from build123d import *

# Parameters (mm, degrees)
SKETCH1_W              = 50
SKETCH1_H              = 50
BOSS_EXTRUDE1_DEPTH    = 6.35
SKETCH6_W              = 25.4
SKETCH6_H              = 25.4
BOSS_EXTRUDE3_DEPTH    = 12.7
SKETCH10_W             = 25.4
SKETCH10_H             = 25.4
CUT_EXTRUDE2_DEPTH     = 15.875
FILLET3_R              = 2.54
SKETCH11_W             = 9.125
SKETCH11_H             = 7.62
BOSS_EXTRUDE4_DEPTH    = 6.35
FILLET4_R              = 2.54
CUT_EXTRUDE3_DEPTH     = 7.35
FILLET4_OF_MIRROR1_R   = 2.54
FILLET5_R              = 2.54
CUT_EXTRUDE4_DEPTH     = 2.54
SKETCH14_R             = 4.7625
CUT_EXTRUDE5_DEPTH     = 16.875
FILLET6_R              = 2.54
F_10_CLEARANCE_HOLE1_D = 5.1054
F_8_CLEARANCE_HOLE1_D  = 4.4958


with BuildPart() as part:
    # Sketch1 → Boss-Extrude1 (new body)
    with BuildSketch(Plane.XY):
        Rectangle(SKETCH1_W, SKETCH1_H)
    extrude(amount=BOSS_EXTRUDE1_DEPTH)

    # Sketch6 → Boss-Extrude3 (add)
    with BuildSketch(Plane.XY.offset(6.35)):
        with BuildLine():
            Line((15.875, 19.05), (15.875, 25))
            Line((15.875, 25), (-15.875, 25))
            Line((-15.875, 25), (-15.875, 19.05))
            ThreePointArc((-15.875, 19.05), (-16.80493597, 16.80493597), (-19.05, 15.875))
            Line((-19.05, 15.875), (-25, 15.875))
            Line((-25, 15.875), (-25, -15.875))
            Line((-25, -15.875), (-19.05, -15.875))
            ThreePointArc((-19.05, -15.875), (-16.80493597, -16.80493597), (-15.875, -19.05))
            Line((-15.875, -19.05), (-15.875, -25))
            Line((-15.875, -25), (15.875, -25))
            Line((15.875, -25), (15.875, -19.05))
            ThreePointArc((15.875, -19.05), (16.80493597, -16.80493597), (19.05, -15.875))
            Line((19.05, -15.875), (25, -15.875))
            Line((25, -15.875), (25, 15.875))
            Line((25, 15.875), (19.05, 15.875))
            ThreePointArc((19.05, 15.875), (16.80493597, 16.80493597), (15.875, 19.05))
        make_face()
        Rectangle(SKETCH6_W, SKETCH6_H, mode=Mode.SUBTRACT)
    extrude(amount=BOSS_EXTRUDE3_DEPTH)

    # Sketch10 → Cut-Extrude2 (cut)
    with BuildSketch(Plane.XY.offset(19.05)):
        Rectangle(SKETCH10_W, SKETCH10_H)
    extrude(amount=-CUT_EXTRUDE2_DEPTH, mode=Mode.SUBTRACT)

    # Fillet3
    fillet3_edges = [part.edges().sort_by_distance(p)[0] for p in [
        (-15.875, -25, 12.7),
        (15.875, -25, 12.7),
        (25, -15.875, 12.7),
        (25, 15.875, 12.7),
        (15.875, 25, 12.7),
        (-15.875, 25, 12.7),
        (-25, 15.875, 12.7),
        (-25, -15.875, 12.7),
    ]]
    fillet(fillet3_edges, radius=FILLET3_R)

    # Sketch11 → Boss-Extrude4 (add)
    with BuildSketch(Plane.XY.offset(6.35)):
        with Locations((20.4375, -28.81)):
            Rectangle(SKETCH11_W, SKETCH11_H)
    boss_extrude4 = extrude(amount=-BOSS_EXTRUDE4_DEPTH)

    # Fillet4
    fillet4_edges = [part.edges().sort_by_distance(p)[0] for p in [
        (25, -32.62, 3.175),
        (15.875, -32.62, 3.175),
    ]]
    fillet(fillet4_edges, radius=FILLET4_R)

    # Sketch12 → Cut-Extrude3 (cut, through all)
    with BuildSketch(Plane.XY.offset(6.35)):
        with BuildLine():
            Line((19.285, -28.575), (19.285, -22.225))
            ThreePointArc((19.285, -22.225), (20.555, -20.955), (21.825, -22.225))
            Line((21.825, -22.225), (21.825, -28.575))
            ThreePointArc((21.825, -28.575), (20.555, -29.845), (19.285, -28.575))
        make_face()
    cut_extrude3 = extrude(amount=-CUT_EXTRUDE3_DEPTH, mode=Mode.SUBTRACT)

    # Mirror1: Boss-Extrude4, Cut-Extrude3 across plane
    add(boss_extrude4.mirror(Plane.ZX))
    add(cut_extrude3.mirror(Plane.ZX), mode=Mode.SUBTRACT)

    # Fillet4 of Mirror1
    fillet4_of_mirror1_edges = [part.edges().sort_by_distance(p)[0] for p in [
        (25, 32.62, 3.175),
        (15.875, 32.62, 3.175),
    ]]
    fillet(fillet4_of_mirror1_edges, radius=FILLET4_OF_MIRROR1_R)

    # Fillet5
    fillet5_edges = [part.edges().sort_by_distance(p)[0] for p in [
        (15.875, -25, 3.175),
        (15.875, 25, 3.175),
        (-25, 25, 3.175),
        (-25, -25, 3.175),
    ]]
    fillet(fillet5_edges, radius=FILLET5_R)

    # Sketch13 → Cut-Extrude4 (cut)
    with BuildSketch(Plane.XY.offset(6.35)):
        with BuildLine():
            Line((22.46, 32.62), (18.415, 32.62))
            ThreePointArc((18.415, 32.62), (16.618948776, 31.876051224), (15.875, 30.08))
            Line((15.875, 30.08), (15.875, 27.54))
            ThreePointArc((15.875, 27.54), (15.131051224, 25.743948776), (13.335, 25))
            ThreePointArc((13.335, 25), (15.131051224, 24.256051224), (15.875, 22.46))
            Line((15.875, 22.46), (15.875, 19.05))
            ThreePointArc((15.875, 19.05), (16.80493597, 16.80493597), (19.05, 15.875))
            Line((19.05, 15.875), (22.46, 15.875))
            ThreePointArc((22.46, 15.875), (24.256051224, 15.131051224), (25, 13.335))
            Line((25, 13.335), (25, 30.08))
            ThreePointArc((25, 30.08), (24.256051224, 31.876051224), (22.46, 32.62))
        make_face()
        with BuildLine():
            Line((15.875, -27.54), (15.875, -30.08))
            ThreePointArc((15.875, -30.08), (16.618948776, -31.876051224), (18.415, -32.62))
            Line((18.415, -32.62), (22.46, -32.62))
            ThreePointArc((22.46, -32.62), (24.256051224, -31.876051224), (25, -30.08))
            Line((25, -30.08), (25, -13.335))
            ThreePointArc((25, -13.335), (24.256051224, -15.131051224), (22.46, -15.875))
            Line((22.46, -15.875), (19.05, -15.875))
            ThreePointArc((19.05, -15.875), (16.80493597, -16.80493597), (15.875, -19.05))
            Line((15.875, -19.05), (15.875, -22.46))
            ThreePointArc((15.875, -22.46), (15.131051224, -24.256051224), (13.335, -25))
            ThreePointArc((13.335, -25), (15.131051224, -25.743948776), (15.875, -27.54))
        make_face()
    extrude(amount=-CUT_EXTRUDE4_DEPTH, mode=Mode.SUBTRACT)

    # Sketch14 → Cut-Extrude5 (cut, through all)
    with BuildSketch(Plane.XY.offset(3.175)):
        with Locations((-10, 0)):
            Circle(SKETCH14_R)
        with Locations((0, -10)):
            Circle(SKETCH14_R)
        with Locations((10, 0)):
            Circle(SKETCH14_R)
        with Locations((0, 10)):
            Circle(SKETCH14_R)
    extrude(amount=CUT_EXTRUDE5_DEPTH, mode=Mode.SUBTRACT)

    # Fillet6
    fillet6_edges = [part.edges().sort_by_distance(p)[0] for p in [
        (-12.7, 3.923188276, 11.1125),
        (-12.7, -3.923188276, 11.1125),
        (-3.923188276, -12.7, 11.1125),
        (3.923188276, -12.7, 11.1125),
        (12.7, 3.923188276, 11.1125),
        (12.7, -3.923188276, 11.1125),
        (-3.923188276, 12.7, 11.1125),
        (3.923188276, 12.7, 11.1125),
    ]]
    fillet(fillet6_edges, radius=FILLET6_R)

    # #10 Clearance Hole1 (through all)
    with Locations(Plane.XY.offset(3.175)):
        with Locations((-10, 0), (0, 10), (10, 0), (0, -10)):
            Hole(F_10_CLEARANCE_HOLE1_D / 2)

    # #8 Clearance Hole1 (through all)
    with Locations(Plane.XY.offset(19.05)):
        with Locations((-19.92, 0), (19.92, 0)):
            Hole(F_8_CLEARANCE_HOLE1_D / 2)


solid = part.part
For this review, take the finished solid that the model builds, in its own axes (mm). A direction names the side the tool comes from. Round coordinates to 2 decimals unless told otherwise and drop trailing zeros. Loops run counter-clockwise (first coordinate to the right, second up) from the corner with the lowest first, then second, coordinate; pieces in that order, holes last. Notation, with made-up numbers: (-12.5, 56.25) - (13.5, 56.25) arc R11 ccw to (13.5, 74.25) - close; hole circle Ø11 at (40, 18). An arc over 180 degrees is marked (long way). Use one line per item in the form item = value.
Item 1: For line 1 (Y direction, x = -19.92, z = 9.5) (3 decimals); line 2 (Y direction, x = -10, z = 1.2); line 3 (X direction, y = -28.5, z = 2) (3 decimals), list the stretches that pass through material, from the lowest coordinate up.
Answers:
line_1 = -15.875 to -2.248, 2.248 to 15.875
line_2 = -25 to -2.55, 2.55 to 25
line_3 = 15.875 to 19.285, 21.825 to 25
Item 2: Consider section C-C on y = 0. State how many separate pieces and enclosed holes the cut face has, then the cut area to 3 significant figures.
Answers:
separate_pieces = 5
enclosed_holes = 0
area = 280 mm^2
Item 3: Tool access review of faces 5 (the flat face through (-21, 21, 6.35)), 6 (the cylindrical face through (-15.151, -24.236, 12.789)), 7 (the cylindrical face through (4.1, 12.9, 11)): name each direction out of +Z, -Z, +X, -X, +Y, -Y from which nothing blocks a thin tool from reaching the whole face with its end or side.
Answers:
face_5 = +Z, -X, +Y
face_6 = +Z, -X, -Y
face_7 = +Z
Item 4: Clearance check with flat-ended pins moving along their axes: P1, Ø5, axis at y = -17.5, z = 8, coming from the +X side; P2, Ø5.5, axis at x = -7.5, z = 12, coming from the -Y side; P3, Ø2.5, axis at x = -21, z = 12, coming from the -Y side (3 decimals); P4, Ø4, axis at x = 19.92, y = 0, coming from the +Z side. State where each tip first meets the part, or that it passes through.
Answers:
P1 = 24.38
P2 = -25
P3 = -15.875
P4 = through
Item 5: Mouldability with a two-part tool opening along X and no side actions: class faces 1 (the flat face through (-15.875, -21, 13)), 2 (the cylindrical face through (24.276, -31.856, 1.878)), 3 (the cylindrical face through (0.553, -12.492, 1.565)), 4 (the cylindrical face through (0.051, 14.762, 11.001)) as +X half, -X half, draft (parallel to the pull), parting line (faces both ways), or undercut.
Answers:
face_1 = -X half
face_2 = +X half
face_3 = undercut
face_4 = undercut
Item 6: Consider section A-A on y = -10. Write out the cut boundary in (x, z) (3 decimals).
Answers:
outline = (-25, 0) - (-2.553, 0) - (-2.553, 3.175) - (-12.7, 3.175) - (-12.7, 19.05) - (-25, 19.05) - close; (2.553, 0) - (25, 0) - (25, 19.05) - (12.7, 19.05) - (12.7, 3.175) - (2.553, 3.175) - close
